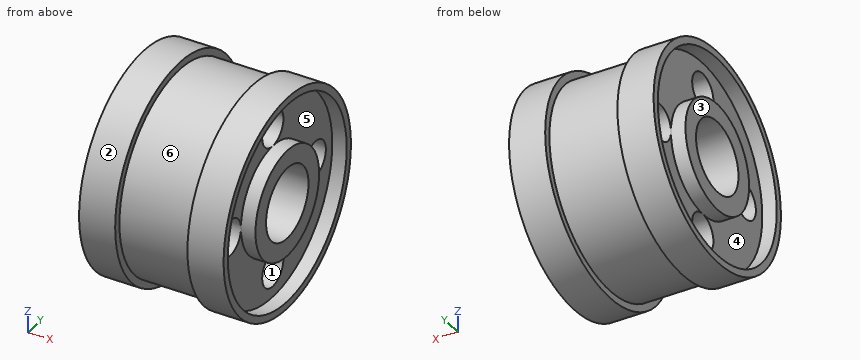
from build123d import *

# Parameters (mm, degrees)
F2_R     = 2.5
F3_DEPTH = 20.001
F5_R     = 14
F5_R_2   = 7.5
F6_DEPTH = 3
F8_R     = 14
F8_R_2   = 7.5
F9_DEPTH = 3


with BuildPart() as f1:
    # F0 (on Top) → F1 (revolve)
    with BuildSketch(Plane.XY):
        Polygon((12.0361039788, 5), (12.0361039788, 15), (7.0361039788, 15), (7.0361039788, 14), (-2.9638960212, 14), (-2.9638960212, 15), (-7.9638960212, 15), (-7.9638960212, 5), align=None)
    revolve(axis=Axis((-2.1188026294, 0, 0), (1, 0, 0)))

    # F2 (on face) → F3 (cut, through all)
    with BuildSketch(Plane(origin=(-7.9638960212, 0, 0), x_dir=(0, -1, 0), z_dir=(-1, 0, 0))):
        with Locations((-10, 0)):
            Circle(F2_R)
        with Locations((10, 0)):
            Circle(F2_R)
        with Locations((0, 10)):
            Circle(F2_R)
        with Locations((0, -10)):
            Circle(F2_R)
    extrude(amount=-F3_DEPTH, mode=Mode.SUBTRACT)

    # F5 (on offset) → F6 (cut)
    with BuildSketch(Plane(origin=(-8.9638960212, 0, 0), x_dir=(0, -1, 0), z_dir=(-1, 0, 0))):
        Circle(F5_R)
        Circle(F5_R_2, mode=Mode.SUBTRACT)
    extrude(amount=-F6_DEPTH, mode=Mode.SUBTRACT)

    # F8 (on offset) → F9 (cut)
    with BuildSketch(Plane.YZ.offset(13.0361039788)):
        Circle(F8_R)
        Circle(F8_R_2, mode=Mode.SUBTRACT)
    extrude(amount=-F9_DEPTH, mode=Mode.SUBTRACT)


solid = f1.part
Verification items for the finished model (mm, model axes). Face numbers are marked on the shaded views. A direction names the side the tool comes from. Round coordinates to 2 decimals unless told otherwise and drop trailing zeros. Loops run counter-clockwise (first coordinate to the right, second up) from the corner with the lowest first, then second, coordinate; pieces in that order, holes last. Notation, with made-up numbers: M -25.75,28.25 L 17.25,28.25 A16 ccw 17.25,57.25 Z; hole C -39.75,-16 d9. An arc over 180 degrees is marked long. Write each question's results on one line, items separated by ' | '.
1) Mould release check, pull along Z, two halves, no side actions. Record for the marked faces 1, 2 and 3: released by +Z, released by -Z, zero draft, split by the parting line, or undercut.
Checks:
face 1: undercut | face 2: split by the parting line | face 3: zero draft
2) Scan lines: L1, parallel to Z at x = 7.25, y = 0; L2, parallel to Z at x = 2.25, y = 0; L3, parallel to X at y = 9, z = -11.75. Record each from-to range of solid material in increasing order. Write a range as from..to.
Checks:
L1: z = -15..-12.5, -7.5..-5, 5..7.5, 12.5..15 | L2: z = -14..-12.5, -7.5..-5, 5..7.5, 12.5..14 | L3: x = -7.96..-2.96, 7.04..12.04
3) Section check A-A on x = 1. Record the boundary of the cut face in (y, z).
Checks:
outline: C 0,0 d28; hole C -10,0 d5; hole C 0,0 d10; hole C 0,-10 d5; hole C 0,10 d5; hole C 10,0 d5
4) Section check C-C on z = -8.75. Record the boundary of the cut face in (x, y), then the cut area to 3 significant figures.
Checks:
outline: M -7.96,-12.18 L -2.96,-12.18 L -2.96,-10.93 L 7.04,-10.93 L 7.04,-12.18 L 12.04,-12.18 L 12.04,-10.93 L 10.04,-10.93 L 10.04,-2.17 L -5.96,-2.17 L -5.96,-10.93 L -7.96,-10.93 Z; M -7.96,10.93 L -5.96,10.93 L -5.96,2.17 L 10.04,2.17 L 10.04,10.93 L 12.04,10.93 L 12.04,12.18 L 7.04,12.18 L 7.04,10.93 L -2.96,10.93 L -2.96,12.18 L -7.96,12.18 Z | area: 306 mm2
5) Access from +Z, -Z, +X, -X, +Y, -Y to the whole of each face (thin tool, end or side, straight path). Record for the marked faces 4, 5 and 6.
Checks:
face 4: -X | face 5: +X | face 6: none
6) Section check D-D on x = -3.5. Record the boundary of the cut face in (y, z), then the cut area to 3 significant figures.
Checks:
outline: C 0,0 d30; hole C -10,0 d5; hole C 0,0 d10; hole C 0,-10 d5; hole C 0,10 d5; hole C 10,0 d5 | area: 550 mm2
7) Section check B-B on y = -10.5. Record the boundary of the cut face in (x, z).
Checks:
outline: M -7.96,-10.71 L -2.96,-10.71 L -2.96,-9.26 L 7.04,-9.26 L 7.04,-10.71 L 12.04,-10.71 L 12.04,-9.26 L 10.04,-9.26 L 10.04,-2.45 L -5.96,-2.45 L -5.96,-9.26 L -7.96,-9.26 Z; M -7.96,9.26 L -5.96,9.26 L -5.96,2.45 L 10.04,2.45 L 10.04,9.26 L 12.04,9.26 L 12.04,10.71 L 7.04,10.71 L 7.04,9.26 L -2.96,9.26 L -2.96,10.71 L -7.96,10.71 Z
8) Gauge pin test, flat ends, axial feed: P1, Ø1.5, axis at x = 2, y = 9.5, coming from the +Z side; P2, Ø1.5, axis at y = 10, z = 3, coming from the +X side; P3, Ø4, axis at x = 3, y = -7, coming from the -Z side. Record the tip position at first contact, or that the pin passes through.
Checks:
P1: stops at z = 10.93 | P2: stops at x = 10.04 | P3: stops at z = -13.08
